from build123d import *

# Parameters (mm, degrees)
F0_R     = 2.0193
F1_DEPTH = 10
F2_W     = 27.966302
F2_H     = 13.370458
F3_DEPTH = 2
F4_DEPTH = 6


with BuildPart() as f1:
    # F0 (on Top) → F1 (new body)
    with BuildSketch(Plane.XY):
        with BuildLine():
            Line((-6.5, -17.5), (6.5, -17.5))
            ThreePointArc((6.5, -17.5), (7.207107, -17.207107), (7.5, -16.5))
            Line((7.5, -16.5), (7.5, 13.5))
            ThreePointArc((7.5, 13.5), (6.328427, 16.328427), (3.5, 17.5))
            Line((3.5, 17.5), (-3.5, 17.5))
            ThreePointArc((-3.5, 17.5), (-6.328427, 16.328427), (-7.5, 13.5))
            Line((-7.5, 13.5), (-7.5, -16.5))
            ThreePointArc((-7.5, -16.5), (-7.207107, -17.207107), (-6.5, -17.5))
        make_face()
        with Locations((0, -13.698686)):
            Circle(F0_R, mode=Mode.SUBTRACT)
        with BuildLine():
            Line((-5, -4.897373), (-5, 4.822578))
            ThreePointArc((-5, 4.822578), (0, 9.822578), (5, 4.822578))
            Line((5, 4.822578), (5, -4.897373))
            ThreePointArc((5, -4.897373), (0, -9.897373), (-5, -4.897373))
        make_face(mode=Mode.SUBTRACT)
        with BuildLine():
            ThreePointArc((5, 4.822578), (0, 9.822578), (-5, 4.822578))
            Line((-5, 4.822578), (-5, -4.897373))
            ThreePointArc((-5, -4.897373), (0, -9.897373), (5, -4.897373))
            Line((5, -4.897373), (5, 4.822578))
        make_face()
        with BuildLine():
            Line((-2.75, -4.897373), (-2.75, 4.822578))
            ThreePointArc((-2.75, 4.822578), (0, 7.572578), (2.75, 4.822578))
            Line((2.75, 4.822578), (2.75, -4.897373))
            ThreePointArc((2.75, -4.897373), (0, -7.647373), (-2.75, -4.897373))
        make_face(mode=Mode.SUBTRACT)
    extrude(amount=F1_DEPTH)

    # F2 (on face) → F3 (cut)
    with BuildSketch(Plane.XY.offset(10)):
        with Locations((-0.129465, 18.378206)):
            Rectangle(F2_W, F2_H)
    extrude(amount=-F3_DEPTH, mode=Mode.SUBTRACT)

    # F0 (on Top) → F4 (cut)
    with BuildSketch(Plane.XY):
        with BuildLine():
            ThreePointArc((5, 4.822578), (0, 9.822578), (-5, 4.822578))
            Line((-5, 4.822578), (-5, -4.897373))
            ThreePointArc((-5, -4.897373), (0, -9.897373), (5, -4.897373))
            Line((5, -4.897373), (5, 4.822578))
        make_face()
        with BuildLine():
            Line((-2.75, -4.897373), (-2.75, 4.822578))
            ThreePointArc((-2.75, 4.822578), (0, 7.572578), (2.75, 4.822578))
            Line((2.75, 4.822578), (2.75, -4.897373))
            ThreePointArc((2.75, -4.897373), (0, -7.647373), (-2.75, -4.897373))
        make_face(mode=Mode.SUBTRACT)
    extrude(amount=F4_DEPTH, mode=Mode.SUBTRACT)


solid = f1.part
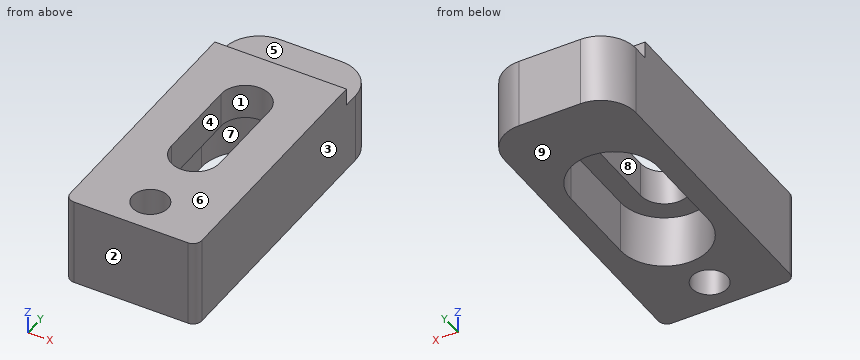
Can you work these out from the model? Positions are in its coordinate system, mm. Face numbers are marked on the shaded views. A direction names the side the tool comes from. Coordinates: 2 decimals unless noted, no trailing zeros. Write each loop counter-clockwise with the first axis right and the second up, starting at its lowest first coordinate (ties: lowest second). Pieces come first, ordered by that corner, then holes. Notation, with made-up numbers: (27, 25.25) -> (38, 25.25) arc R23 cw to (38, 53.25) -> close; hole circle Ø11 at (44, 39.25). An arc over 180 degrees is marked (long way). Write each question's results on one line, items separated by ' | '. Start each with the question number.
Q1. Imagine slicing it at B-B (y = -2.5). Write out the boundary of the cut face in (x, z), then the cut area to 3 significant figures.
Q2. We'd pull the mould along Y, two halves only. Please class the marked faces 1, 2, 3 and 4: +Y half, -Y half, draft (parallel to the pull), parting line (faces both ways), or undercut.
Q3. Imagine slicing it at D-D (x = 4). Write out the boundary of the cut face in (y, z), then the cut area to 3 significant figures.
Q4. Imagine slicing it at A-A (x = 0). Write out the boundary of the cut face in (y, z), then the cut area to 3 significant figures.
Q5. Imagine slicing it at C-C (z = 7.5). Write out the boundary of the cut face in (x, y), then the cut area to 3 significant figures.
Q6. On a 3-axis mill with a long thin cutter (end or side, diameter ignored), from which of +Z, -Z, +X, -X, +Y, -Y can I reach the whole of each face in a straight line? I mean the marked faces 5, 6, 7, 8 and 9. Say none if no direction works.
Q7. If I drill on probe 1 along Y at (x, z) = (0, 5); probe 2 along X at (y, z) = (4, 3.75); probe 3 along X at (y, z) = (-2, 9.75), over which ranges is the centre line in solid material (lowest first)?
Q8. I'm going to push a flat-ended pin straight in: pin 1 (3 mm diameter, centred on x = -1.5, y = 14, fed in from +Z). Where does the tip first touch, or does it pass through?
Taken from the geometry:
1) outline: (-7.5, 0) -> (-5, 0) -> (-5, 6) -> (-2.75, 6) -> (-2.75, 10) -> (-7.5, 10) -> close; (2.75, 6) -> (5, 6) -> (5, 0) -> (7.5, 0) -> (7.5, 10) -> (2.75, 10) -> close | area: 68.0 mm^2
2) face 1: undercut | face 2: -Y half | face 3: draft | face 4: undercut
3) outline: (-17.5, 0) -> (-7.9, 0) -> (-7.9, 6) -> (7.82, 6) -> (7.82, 0) -> (17.47, 0) -> (17.47, 8) -> (11.69, 8) -> (11.69, 10) -> (-17.5, 10) -> close | area: 244 mm^2
4) outline: (-17.5, 0) -> (-15.72, 0) -> (-15.72, 10) -> (-17.5, 10) -> close; (-11.68, 0) -> (-9.9, 0) -> (-9.9, 6) -> (-7.65, 6) -> (-7.65, 10) -> (-11.68, 10) -> close; (7.57, 6) -> (9.82, 6) -> (9.82, 0) -> (17.5, 0) -> (17.5, 8) -> (11.69, 8) -> (11.69, 10) -> (7.57, 10) -> close | area: 119 mm^2
5) outline: (-7.5, -16.5) arc R1 ccw to (-6.5, -17.5) -> (6.5, -17.5) arc R1 ccw to (7.5, -16.5) -> (7.5, 13.5) arc R4 ccw to (3.5, 17.5) -> (-3.5, 17.5) arc R4 ccw to (-7.5, 13.5) -> close; hole (-2.75, -4.9) arc R2.75 ccw to (2.75, -4.9) -> (2.75, 4.82) arc R2.75 ccw to (-2.75, 4.82) -> close; hole circle Ø4.04 at (0, -13.7) | area: 428 mm^2
6) face 5: +Z, +X, -X, +Y | face 6: +Z, +X, -X, +Y, -Y | face 7: -Z | face 8: +Z, -Z | face 9: -Z, +X, -X, +Y, -Y
7) probe 1: y = -17.5 to -15.72, -11.68 to -9.9, 9.82 to 17.5 | probe 2: x = -7.5 to -5, 5 to 7.5 | probe 3: x = -7.5 to -2.75, 2.75 to 7.5
8) pin 1: stops at z = 8
